from build123d import *

# Parameters (mm, degrees)
F0_W     = 25.4
F0_H     = 25.4
F1_DEPTH = 6.35
F3_DEPTH = 2.54
F4_W     = 6.35
F4_H     = 25.4
F5_DEPTH = 25.4010001
F7_DEPTH = 2.5410001
F9_DEPTH = 2.5410001


with BuildPart() as f1:
    # F0 (on Front) → F1 (new body)
    with BuildSketch(Plane.XZ):
        Rectangle(F0_W, F0_H)
    extrude(amount=F1_DEPTH)

    # F2 (on face) → F3 (join)
    with BuildSketch(Plane.XZ.offset(6.35)):
        with BuildLine():
            add(Edge.make_bspline(
                [(0, 12.0295938104), (-0.3149582598, 11.5638402948), (-1.1067667998, 10.3929308176), (-1.116096827, 7.8107129391), (-1.1217156425, 6.2556257471)],
                knots=[0, 0, 0, 0, 0.3977707284, 1, 1, 1, 1], degree=3))
            Line((-1.1217156425, 6.2556257471), (-2.3930480238, 4.719432909))
            Line((-2.3930480238, 4.719432909), (-2.3930480238, 1.329213148))
            Line((-2.3930480238, 1.329213148), (-8.7497094646, -4.4977269135))
            Line((-8.7497094646, -4.4977269135), (-8.7497094646, -5.5571701378))
            Line((-8.7497094646, -5.5571701378), (-7.902154699, -6.7225582898))
            Line((-7.902154699, -6.7225582898), (-3.7173526362, -7.9938909039))
            Line((-3.7173526362, -7.9938909039), (-5.6243510917, -10.0068338215))
            Line((-5.6243510917, -10.0068338215), (-5.6243510917, -11.4370826632))
            Line((-5.6243510917, -11.4370826632), (-3.7173526362, -12.2316647321))
            Line((-3.7173526362, -12.2316647321), (-1.1217156425, -10.4835834354))
            Line((-1.1217156425, -10.4835834354), (-1.1217156425, -9.4241397455))
            Line((-1.1217156425, -9.4241397455), (1.1217156425, -9.4241397455))
            Line((1.1217156425, -9.4241397455), (1.1217156425, -10.4835834354))
            Line((1.1217156425, -10.4835834354), (3.7173526362, -12.2316647321))
            Line((3.7173526362, -12.2316647321), (5.6243510917, -11.4370826632))
            Line((5.6243510917, -11.4370826632), (5.6243510917, -10.0068338215))
            Line((5.6243510917, -10.0068338215), (3.7173526362, -7.9938909039))
            Line((3.7173526362, -7.9938909039), (7.902154699, -6.7225582898))
            Line((7.902154699, -6.7225582898), (8.7497094646, -5.5571701378))
            Line((8.7497094646, -5.5571701378), (8.7497094646, -4.4977269135))
            Line((8.7497094646, -4.4977269135), (2.3930480238, 1.329213148))
            Line((2.3930480238, 1.329213148), (2.3930480238, 4.719432909))
            Line((2.3930480238, 4.719432909), (1.1217156425, 6.2556257471))
            add(Edge.make_bspline(
                [(0, 12.0295938104), (0.3149582598, 11.5638402948), (1.1067667998, 10.3929308176), (1.116096827, 7.8107129391), (1.1217156425, 6.2556257471)],
                knots=[0, 0, 0, 0, 0.3977707284, 1, 1, 1, 1], degree=3))
        make_face()
    extrude(amount=F3_DEPTH)

    # F4 (on face) → F5 (cut, through all)
    with BuildSketch(Plane.YZ.offset(12.7)):
        with Locations((-3.175, 0)):
            Rectangle(F4_W, F4_H)
    extrude(amount=-F5_DEPTH, mode=Mode.SUBTRACT)

    # F6 (on face) → F7 (cut, through all)
    with BuildSketch(Plane.XZ.offset(8.89)):
        Polygon((-3.7173526362, -7.9938909039), (-5.6243510917, -10.0068338215), (-3.7173526362, -8.3735641092), align=None)
    extrude(amount=-F7_DEPTH, mode=Mode.SUBTRACT)

    # F8 (on face) → F9 (cut, through all)
    with BuildSketch(Plane.XZ.offset(8.89)):
        Polygon((3.7173526362, -8.4037045017), (5.6243510917, -10.0068338215), (3.7173526362, -7.9938909039), align=None)
    extrude(amount=-F9_DEPTH, mode=Mode.SUBTRACT)


solid = f1.part
Could you check a few things on this model? Use its own coordinates, in mm. A direction names the side the tool comes from. Coordinates: 2 decimals unless noted, no trailing zeros. Order: outer loops, then holes, each group sorted by start corner. A loop starts at its lowest first (then second) coordinate and runs counter-clockwise, first axis right, second up.
Q1. Which directions (+Z, -Z, +X, -X, +Y, -Y) give clear straight access to the entire face, cutting with the end or side of a thin tool? Please do faces 1 (the flat face through (-1.122, -8, -10)), 2 (the flat face through (5.78, -7.602, -7.367)), 3 (the flat face through (-5.624, -8, -11)).
Q2. Will these pins go through, and if not, where does the flat tip stop? pin 1 (0.7 mm diameter, centred on y = -7.5, z = -11, fed in from +X); pin 2 (1.3 mm diameter, centred on y = -7, z = 2.5, fed in from +X).
Q3. Suppose I cut it at C-C on z = -3.75. Please give me the cut outline in (x, y).
Q4. Suppose I cut it at A-A on x = -5.25. Please give me the cut outline in (y, z).
Q5. Thinking about a two-plate mould opening in Z: for faces 4 (the flat face through (-5.84, -7.6, -7.35)), 5 (the flat face through (4.66, -7.6, -11.84)), 6 (the flat face through (-5.527, -7.602, -1.543)), 7 (the flat face through (0, -8.89, -3)), which applies, released by +Z, released by -Z, zero draft, split by the parting line, or undercut?
Q6. Please list where these lines run through material, in increasing order: L1, parallel to X at y = -7.4, z = 4; L2, parallel to X at y = -7.55, z = 6.5; L3, parallel to Z at x = -5.5, y = -7.9.
Q7. Suppose I cut it at B-B on x = 7. Please give me the cut outline in (y, z).
Answer:
1. face 1: -Z, +Y, -Y
1. face 2: +X, +Y, -Y
1. face 3: -Z, -X, +Y, -Y
2. pin 1: stops at x = 5.62
2. pin 2: stops at x = 2.39
3. outline: (-7.93, -8.89) - (7.93, -8.89) - (7.93, -6.35) - (-7.93, -6.35) - close
4. outline: (-8.89, -11.59) - (-6.35, -11.59) - (-6.35, -9.69) - (-8.89, -9.69) - close; (-8.89, -7.53) - (-6.35, -7.53) - (-6.35, -1.29) - (-8.89, -1.29) - close
5. face 4: undercut
5. face 5: released by -Z
5. face 6: released by +Z
5. face 7: zero draft
6. L1: x = -2.39 to 2.39
6. L2: x = -1.12 to 1.12
6. L3: z = -11.49 to -9.9, -7.45 to -1.52
7. outline: (-8.89, -7) - (-6.35, -7) - (-6.35, -2.89) - (-8.89, -2.89) - close
